from build123d import *

# Parameters (mm, degrees)
F0_R          = 35
F0_R_2        = 25
F2_DEPTH      = 5
F2_DEPTH_BACK = 5
F1_R          = 25
F1_R_2        = 3.1
F1_R_3        = 11.2
F3_DEPTH      = 3.5
F3_DEPTH_BACK = 3.5
F4_R          = 0.5


with BuildPart() as f2:
    # F0 (on Top) → F2 (new body, two sides)
    with BuildSketch(Plane.XY) as f2_sk:
        Circle(F0_R)
        Circle(F0_R_2, mode=Mode.SUBTRACT)
    extrude(amount=F2_DEPTH)
    extrude(f2_sk.sketch, amount=-F2_DEPTH_BACK)

    # F1 (on Top) → F3 (join, two sides)
    with BuildSketch(Plane.XY) as f3_sk:
        Circle(F1_R)
        with Locations((-11.558051, -12.506845)):
            Circle(F1_R_2, mode=Mode.SUBTRACT)
        with Locations((-5.692771, -18.02711)):
            Circle(F1_R_2, mode=Mode.SUBTRACT)
        with Locations((-17.940855, -5.951534)):
            Circle(F1_R_2, mode=Mode.SUBTRACT)
        with Locations((0, -21.25873)):
            Circle(F1_R_2, mode=Mode.SUBTRACT)
        with Locations((5.951534, -17.940855)):
            Circle(F1_R_2, mode=Mode.SUBTRACT)
        with Locations((0, -14.855075)):
            Circle(F1_R_2, mode=Mode.SUBTRACT)
        with Locations((12.506845, -11.558051)):
            Circle(F1_R_2, mode=Mode.SUBTRACT)
        with Locations((18.02711, -5.692771)):
            Circle(F1_R_2, mode=Mode.SUBTRACT)
        with Locations((-21.25873, 0)):
            Circle(F1_R_2, mode=Mode.SUBTRACT)
        with Locations((-14.855075, 0)):
            Circle(F1_R_2, mode=Mode.SUBTRACT)
        with Locations((-18.02711, 5.692771)):
            Circle(F1_R_2, mode=Mode.SUBTRACT)
        with Locations((-12.506845, 11.558051)):
            Circle(F1_R_2, mode=Mode.SUBTRACT)
        with Locations((-5.951534, 17.940855)):
            Circle(F1_R_2, mode=Mode.SUBTRACT)
        Circle(F1_R_3, mode=Mode.SUBTRACT)
        with Locations((14.855075, 0)):
            Circle(F1_R_2, mode=Mode.SUBTRACT)
        with Locations((17.940855, 5.951534)):
            Circle(F1_R_2, mode=Mode.SUBTRACT)
        with Locations((21.25873, 0)):
            Circle(F1_R_2, mode=Mode.SUBTRACT)
        with Locations((0, 14.855075)):
            Circle(F1_R_2, mode=Mode.SUBTRACT)
        with Locations((5.692771, 18.02711)):
            Circle(F1_R_2, mode=Mode.SUBTRACT)
        with Locations((11.558051, 12.506845)):
            Circle(F1_R_2, mode=Mode.SUBTRACT)
        with Locations((0, 21.25873)):
            Circle(F1_R_2, mode=Mode.SUBTRACT)
    extrude(amount=F3_DEPTH)
    extrude(f3_sk.sketch, amount=-F3_DEPTH_BACK)

    # F4
    f4_edges = [f2.edges().sort_by_distance(p)[0] for p in [
        (35, 0, 2.5),
        (-35, 0, 0),
        (-35, 0, 5),
    ]]
    fillet(f4_edges, radius=F4_R)


solid = f2.part
Verification items for the finished model (mm, model axes). A direction names the side the tool comes from. Give positions to 0.01 mm unless a question says otherwise; leave off trailing zeros.
1. Material ranges on probe 1 along X at (y, z) = (-12.5, -2); probe 2 along X at (y, z) = (-6, 2); probe 3 along Y at (x, z) = (-1, -2.5), recorded low to high.
Derived:
probe 1: x = -32.69 to -14.66, -8.46 to -2.02, 2.02 to 9.55, 15.46 to 32.69
probe 2: x = -34.48 to -21.04, -14.84 to -9.46, 9.46 to 14.94, 21.11 to 34.48
probe 3: y = -34.99 to -24.19, -18.32 to -17.79, -11.92 to -11.16, 11.16 to 11.92, 17.79 to 18.32, 24.19 to 34.99
2. Go/stop test with flat-tipped pins: P1, Ø5, axis at x = 19, z = 0, coming from the +Y side; P2, Ø5, axis at x = -21.26, y = 0, coming from the +Z side; P3, Ø1, axis at y = -8, z = -3.5, coming from the -X side; P4, Ø10, axis at x = -11.56, y = -12.51, coming from the -Z side. Record where each tip stops, or that it passes through.
Derived:
P1: stops at y = 30.87
P2: passes through
P3: stops at x = -34.19
P4: stops at z = -3.5
3. Tool access check on faces 5 (the flat face through (18, 18, -5)), 6 (the flat face through (5, -11, 3.5)). Record the directions out of +Z, -Z, +X, -X, +Y, -Y that give a thin tool (end or side, any length) a straight path to the whole face; none if there is none.
Derived:
face 5: -Z, +X, -X, +Y, -Y
face 6: +Z
4. Cross-section at A-A on z = -1.25. Count the separate pieces of the cut face and the enclosed holes in it, and give its area (3 significant figures).
Derived:
separate pieces: 1
enclosed holes: 21
area: 2,850 mm2
5. Release check for a two-part mould opening along X. For faces 1 (the flat face through (5, -11, -3.5)), 2 (the cylindrical face through (23.846, 7.509, -4.24)), 3 (the cylindrical face through (-28, -21, 0)), 4 (the flat face through (18, 18, 5)) record: +X half, -X half, draft (parallel to the pull), parting line (faces both ways), or undercut.
Derived:
face 1: undercut
face 2: undercut
face 3: parting line
face 4: draft
